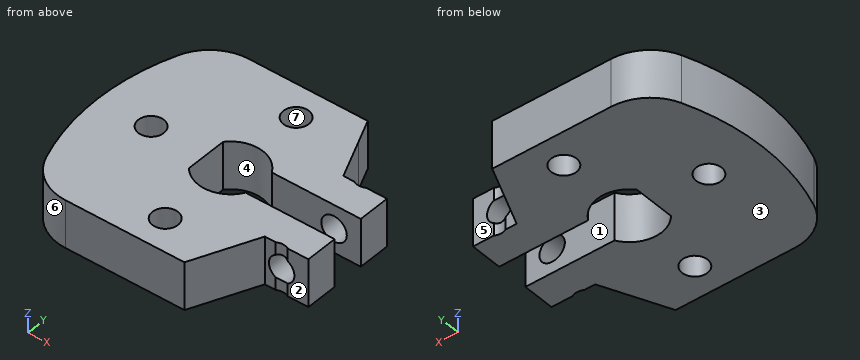
Autodesk Inventor part; units mm, degrees
ref_plane "YZ Plane" through (0, 0, 0) normal (1, 0, 0) x (0, 1, 0)
ref_plane "XZ Plane" through (0, 0, 0) normal (0, 1, 0) x (-1, 0, 0)
ref_plane "XY Plane" through (0, 0, 0) normal (0, 0, 1) x (1, 0, 0)
sketch "スケッチ1" plane through (0, 0, 0) normal (0, 0, 1) x (1, 0, 0)
  line L0 (9, 0) -> (9, 4)
  line L1 (9, 12) -> (2.2731, 12)
  line L2 (0, 8) -> (9, 8)
  line L3 (0, 4) -> (9, 4)
  line L4 (9, 8) -> (9, 12)
  line L5 (2.2731, 12) -> (0, 14.2779)
  line L6 (2.2731, 0) -> (-5.7099, -8)
  line L7 (-5.7099, 20) -> (-15.7099, 20)
  line L8 (-5.7099, -8) -> (-15.7099, -8)
  line L9 (-15.7099, 20) -> (-25.7698, 20)
  line L10 (-25.7698, 20) -> (-25.7698, -8)
  line L11 (-25.7698, -8) -> (-15.7099, -8)
  line L12 (2.2731, 0) -> (9, 0)
  line L13 (0, 14.2779) -> (-5.7099, 20)
  arc A0 (-2.1881, 8) -> (-8.8099, 8.6062) centre (-5.7099, 6) ccw
  line L14 (0, 8) -> (-2.1881, 8)
  line L15 (0, 4) -> (-2.1881, 4)
  line L16 (-8.8099, 8.6062) -> (-8.8099, 3.3938)
  arc A1 (-8.8099, 3.3938) -> (-2.1881, 4) centre (-5.7099, 6) ccw
  point P0 (0, 0)
  point P1 (4.5, 12)
  point P2 (4.5, 0)
  point P3 (4.5, 4)
  point P4 (-25.7099, 6)
  point P5 (-8.8099, 6)
  dimension "d5" = 4
  dimension "d8" = 10
  dimension "d9" = 10
  dimension "d12" = 14
  dimension "d90" = 8.1
  dimension "d91" = 3.1
extrude "押し出し1" add sketch "スケッチ1" along normal blind 6
sketch "スケッチ2" plane through (0, 0, 6) normal (0, 0, 1) x (1, 0, 0)
  circle A0 centre (5.6365, 13.3) radius 1.5
  line L0 (9, 8) -> (9, 12)
  line L1 (11.5477, 6) -> (-28.1936, 6) construction
  line L2 (9, 12) -> (2.2731, 12)
  circle A1 centre (5.6365, -1.3) radius 1.5
  point P0 (0, 0)
  point P1 (4.8882, 12)
  point P2 (6.3849, 12)
  dimension "d15" = 3
  dimension "d16" = 3.3635
  dimension "d17" = 1.3
extrude "押し出し2" cut sketch "スケッチ2" against normal blind 6 contours A0 L2 | A1 picked at (5.4614, 13.0013)
sketch "スケッチ3" plane through (0, 0, 6) normal (0, 0, 1) x (1, 0, 0)
  circle A0 centre (5.6365, 13.3) radius 1.5
  line L0 (9, 12) -> (2.2731, 12)
  point P0 (0, 0)
  point P1 (4.8882, 12)
  point P2 (6.3849, 12)
  dimension "d20" = 3
  dimension "d21" = 1.3
extrude "押し出し3" add sketch "スケッチ3" against normal blind 6 contours A0 L0 picked at (5.4614, 13.0013)
sketch "スケッチ4" plane through (0, 0, 6) normal (0, 0, 1) x (1, 0, 0)
  arc A0 (6.3849, 12) -> (4.8882, 12) centre (5.6365, 13.3) ccw
  circle A1 centre (5.6365, 13.3) radius 1.5
  point P0 (0, 0)
  dimension "d24" = 3
extrude "押し出し4" cut sketch "スケッチ4" against normal blind 6
fillet "フィレット1" radius 5 1 edges at (-25.7698, 20, 3)
fillet "フィレット2" radius 5 1 edges at (-25.7698, -8, 3)
fillet "フィレット3" radius 3 4 edges at (-5.7099, -8, 3) (2.2731, 0, 3) (-5.7099, 20, 3) (2.2731, 12, 3)
sketch "スケッチ6" plane through (0, 4, 0) normal (0, 1, 0) x (1, 0, 0)
  point P0 (0, 0)
sketch "スケッチ7" plane through (4.8882, 12, 6) normal (0, 1, 0) x (1, 0, 0)
  circle A0 centre (0.7488, 3) radius 1.6
  line L0 (1.4967, 0) -> (0, 0)
  line L1 (4.1118, 6) -> (4.1118, 0)
  point P0 (-4.8882, 6)
  point P1 (0.7483, 0)
  dimension "d43" = 3.2
  dimension "d44" = 3
  dimension "d45" = 3.363
extrude "押し出し5" cut sketch "スケッチ7" against normal blind 28
sketch "スケッチ11" plane through (0, 0, 6) normal (0, 0, 1) x (1, 0, 0)
  line L0 (-6.9544, 20) -> (-20.7698, 20)
  line L1 (-20.7698, 20) -> (-6.9544, 20)
  arc A0 (1.394, 12.8809) -> (3.5176, 12) centre (3.5176, 15) ccw
  line L2 (0, 20) -> (1.3068, 17.0279)
  arc A1 (1.394, 12.8809) -> (3.5176, 12) centre (3.5176, 15) ccw
  arc A2 (-4.8308, 19.1191) -> (-6.9544, 20) centre (-6.9544, 17) ccw
  arc A3 (-4.8308, 19.1191) -> (-6.9544, 20) centre (-6.9544, 17) ccw
  line L3 (1.394, 12.8809) -> (-4.8308, 19.1191)
  line L4 (-4.8308, 19.1191) -> (1.394, 12.8809)
  arc A4 (0, 8) -> (0, 4) centre (-5.7099, 6) ccw
  line L5 (-11.7599, 6) -> (12.1155, 6) construction
  line L6 (-20.7698, -8) -> (0, -8)
  line L7 (0, -8) -> (3.5176, 0)
  arc A5 (-6.9544, -8) -> (-4.8308, -7.1191) centre (-6.9544, -5) ccw
  line L8 (1.394, -0.8809) -> (-4.8308, -7.1191)
  line L9 (-6.9544, 20) -> (0, 20)
  line L10 (1.3068, 17.0279) -> (3.5176, 12)
  arc A6 (3.5176, 0) -> (1.394, -0.8809) centre (3.5176, -3) ccw
  point P0 (0, 0)
extrude "押し出し6" add sketch "スケッチ11" against normal blind 6
sketch "スケッチ12" plane through (0, 0, 6) normal (0, 0, 1) x (1, 0, 0)
  arc A0 (0, 8) -> (0, 4) centre (-5.7099, 6) ccw
  point P0 (0, 0)
  point P1 (-15.7099, 6)
  point P2 (-5.7099, 16)
  point P3 (-5.7099, -4)
  dimension "d74" = 10
  dimension "d76" = 10
  dimension "d77" = 10
hole "穴4" at (-15.7099, 6, 6) at (-5.7099, 16, 6) at (-5.7099, -4, 6) direction (0, 0, -1) diameter 3.2 end through all
sketch "スケッチ13" plane through (0, 0, 6) normal (0, 0, 1) x (1, 0, 0)
  line L0 (-20.7698, -8) -> (0, -8)
  line L1 (0, 20) -> (-20.7698, 20)
  line L2 (-18.7698, 20) -> (-18.7698, -8) construction
  line L3 (-25.7698, 15) -> (-25.7698, -3)
  arc A0 (-18.7698, 20) -> (-18.7698, -8) centre (6.3784, 6) ccw
  line L4 (-18.7698, 20) -> (-29.3351, 20)
  line L5 (-29.3351, 20) -> (-29.3351, -8)
  line L6 (-29.3351, -8) -> (-18.7698, -8)
  point P0 (0, 0)
  dimension "d85" = 7
extrude "押し出し7" cut sketch "スケッチ13" against normal blind 6
fillet "フィレット4" radius 6 1 edges at (-18.7698, 20, 3)
fillet "フィレット5" radius 6 1 edges at (-18.7698, -8, 3)
properties part number "射出_腕固定3_真" material "ポリカーボネート、クリア"
Model file for the job. Use its own axes, mm. Face numbers are marked on the shaded views. A direction names the side the tool comes from. Round coordinates to 2 decimals unless told otherwise and drop trailing zeros. Order: outer loops, then holes, each group sorted by start corner. A loop starts at its lowest first (then second) coordinate and runs counter-clockwise, first axis right, second up.
(1) Band-saw the part on C-C (x = 3). List the corners of the cut face in (y, z).
(2) Band-saw the part on B-B (z = 4). List the corners of the cut face in (x, y), then the cut area to 3 significant figures.
(3) Band-saw the part on D-D (x = -19). List the corners of the cut face in (y, z).
(4) Pin check, flat tips, straight feed: pin 1 (1.5 mm diameter, centred on x = 4, z = 2.5, fed in from -Y); pin 2 (1.8 mm diameter, centred on x = 4.5, z = 3, fed in from +Y); pin 3 (1.3 mm diameter, centred on x = 8, z = 2, fed in from -Y). Stop position of each tip, or through.
(5) Band-saw the part on A-A (y = 6). List the corners of the cut face in (x, z).
(6) Pull direction X, two halves, no side cores. Call the marked faces 4, 5, 6 and 7: released by +X, released by -X, zero draft, split by the parting line, or undercut.
(7) Drill centre lines: line 1 (Y direction, x = 4, z = 3.25); line 2 (X direction, y = 9.25, z = 3); line 3 (X direction, y = 6, z = 4). Where is each one in solid material? Low to high.
(8) 3-axis set-ups, long thin cutter, end or side, ignore diameter. For the marked faces 1, 2 and 3: which of +Z, -Z, +X, -X, +Y, -Y reach the whole face in a straight line?
Verdict:
1. outline: (-1.18, 0) - (4, 0) - (4, 6) - (-1.18, 6) - close; (8, 0) - (13.18, 0) - (13.18, 6) - (8, 6) - close
2. outline: (-20.57, -4.11) arc R6 ccw to (-14.95, -8) - (0, -8) - (3.52, 0) - (4.39, 0) - (4.39, 4) - (-2.19, 4) arc R4.05 cw to (-8.81, 3.39) - (-8.81, 8.61) arc R4.05 cw to (-2.19, 8) - (4.39, 8) - (4.39, 12) - (3.52, 12) - (1.31, 17.03) - (0, 20) - (-14.95, 20) arc R6 ccw to (-20.57, 16.11) arc R28.78 ccw to start; (6.89, 0) - (9, 0) - (9, 4) - (6.89, 4) - close; (6.89, 8) - (9, 8) - (9, 12) - (6.89, 12) - close; hole circle Ø3.2 at (-15.71, 6); hole circle Ø3.2 at (-5.71, -4); hole circle Ø3.2 at (-5.71, 16)
2. area: 589 mm2
3. outline: (-6.43, 0) - (18.43, 0) - (18.43, 6) - (-6.43, 6) - close
4. pin 1: stops at y = -0.61
4. pin 2: stops at y = 12
4. pin 3: stops at y = 0
5. outline: (-22.4, 0) - (-17.31, 0) - (-17.31, 6) - (-22.4, 6) - close; (-14.11, 0) - (-8.81, 0) - (-8.81, 6) - (-14.11, 6) - close
6. face 4: undercut
6. face 5: zero draft
6. face 6: released by -X
6. face 7: undercut
7. line 1: y = 0 to 4, 8 to 12
7. line 2: x = -22.22 to -8.13, -3.29 to 4.04, 7.24 to 9
7. line 3: x = -22.4 to -17.31, -14.11 to -8.81
8. face 1: +Z, -Z, +X
8. face 2: +Z, -Z, +X, -Y
8. face 3: -Z, +X, -X, +Y, -Y
